Work out the finished part from the listing and answer in its coordinate system (mm). Give positions to 0.01 mm unless a question says otherwise; leave off trailing zeros. Order: outer loops, then holes, each group sorted by start corner. A loop starts at its lowest first (then second) coordinate and runs counter-clockwise, first axis right, second up. Notation, with made-up numbers: M 3,82 L 23,82 A29 ccw 23,118 Z; hole C -37.5,52 d4. An arc over 180 degrees is marked long. One line per item, written item: value.
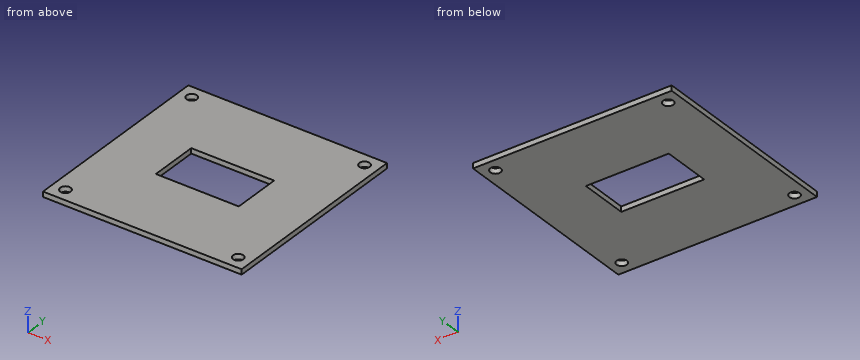
from build123d import *

# Parameters (mm, degrees)
SKETCH_W        = 115
SKETCH_H        = 115
PAD_DEPTH       = 3
SKETCH001_W     = 48
SKETCH001_H     = 28
POCKET_DEPTH    = 5
SKETCH003_R     = 3
POCKET001_DEPTH = 5


with BuildPart() as part:
    # Sketch → Pad (new body)
    with BuildSketch(Plane.XY):
        Rectangle(SKETCH_W, SKETCH_H)
    extrude(amount=PAD_DEPTH)

    # Sketch001 (on Face6 of Pad) → Pocket (cut)
    with BuildSketch(Plane.XY.offset(3)):
        Rectangle(SKETCH001_W, SKETCH001_H)
    extrude(amount=-POCKET_DEPTH, mode=Mode.SUBTRACT)

    # Sketch003 (on Face5 of Pocket) → Pocket001 (cut)
    with BuildSketch(Plane.XY.offset(3)):
        with Locations((50, -50)):
            Circle(SKETCH003_R)
        with Locations((-50, -50)):
            Circle(SKETCH003_R)
        with Locations((-50, 50)):
            Circle(SKETCH003_R)
        with Locations((50, 50)):
            Circle(SKETCH003_R)
    extrude(amount=-POCKET001_DEPTH, mode=Mode.SUBTRACT)


solid = part.part
(1) Section D-D, the plane y = 50 is taken. Give the vertices of the cut face in (x, z), then the cut area to 3 significant figures.
Findings:
outline: M -57.5,0 L -53,0 L -53,3 L -57.5,3 Z; M -47,0 L 47,0 L 47,3 L -47,3 Z; M 53,0 L 57.5,0 L 57.5,3 L 53,3 Z
area: 309 mm^2
(2) Section C-C, the plane z = 1 is taken. Give the vertices of the cut face in (x, y).
Findings:
outline: M -57.5,-57.5 L 57.5,-57.5 L 57.5,57.5 L -57.5,57.5 Z; hole C -50,-50 d6; hole C -50,50 d6; hole M -24,-14 L 24,-14 L 24,14 L -24,14 Z; hole C 50,-50 d6; hole C 50,50 d6
(3) Given P1, Ø5.5, axis at x = -50, y = 50, coming from the -Z side (3 decimals), flat-ended and moving along its own axis, determine where the tip first touches the part or whether it passes through.
Findings:
P1: passes through
(4) Section B-B, the plane x = 14.5 is taken. Give the vertices of the cut face in (y, z), then the cut area to 3 significant figures.
Findings:
outline: M -57.5,0 L -14,0 L -14,3 L -57.5,3 Z; M 14,0 L 57.5,0 L 57.5,3 L 14,3 Z
area: 261 mm^2
(5) Section A-A, the plane y = 10 is taken. Give the vertices of the cut face in (x, z), then the cut area to 3 significant figures.
Findings:
outline: M -57.5,0 L -24,0 L -24,3 L -57.5,3 Z; M 24,0 L 57.5,0 L 57.5,3 L 24,3 Z
area: 201 mm^2
(6) Find the intervals of material crossed by probe 1 along Y at (x, z) = (50, 1.75); probe 2 along Y at (x, z) = (-9.5, 0.75); probe 3 along X at (y, z) = (-49.5, 2.3), in increasing order. Write a range as from..to.
Findings:
probe 1: y = -57.5..-53, -47..47, 53..57.5
probe 2: y = -57.5..-14, 14..57.5
probe 3: x = -57.5..-52.96, -47.04..47.04, 52.96..57.5
